Check sheet for the drawn part. Datum: minimum x, y, z corner. Units: mm. Round coordinates to 2 decimals unless told otherwise and drop trailing zeros. Write each loop counter-clockwise with the first axis right and the second up, starting at its lowest first coordinate (ties: lowest second). Pieces come first, ordered by that corner, then holes.
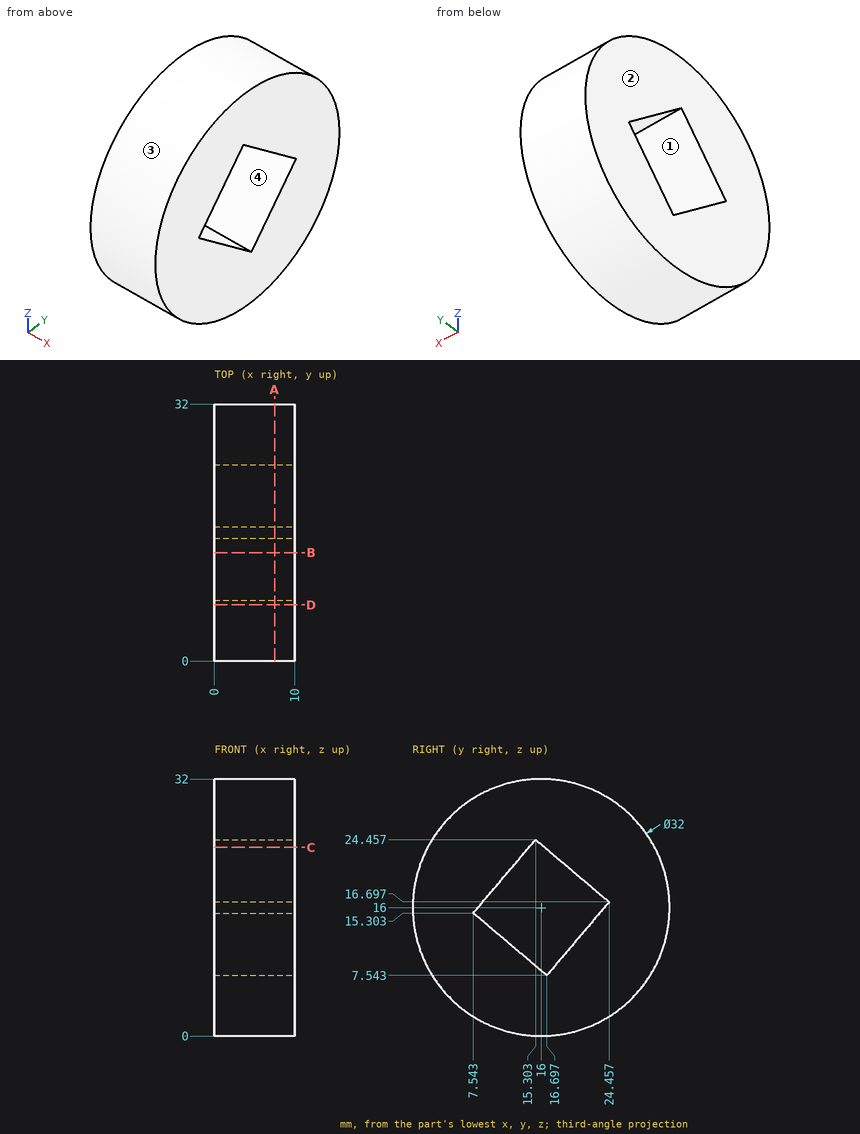
Q1. Sectioned sample at B-B (y = 13.5). Enter the section's corners in (x, z), plus the area to 3 significant figures.
Recorded:
outline: (0, 0.2) - (10, 0.2) - (10, 10.25) - (0, 10.25) - close; (0, 22.33) - (10, 22.33) - (10, 31.8) - (0, 31.8) - close
area: 195 mm2
Q2. Depth check by flat-ended pin: P1, Ø1.5, axis at x = 6.5, z = 10, coming from the +Y side; P2, Ø4, axis at x = 9, z = 12.5, coming from the -Y side; P3, Ø3, axis at x = 1.5, y = 23.5, coming from the +Z side; P4, Ø1, axis at y = 14.5, z = 11.5, coming from the +X side. Enter the tip coordinate at first touch or a pass-through.
Recorded:
P1: stops at y = 31.11
P2: stops at y = 0.07
P3: stops at z = 30.83
P4: passes through
Q3. Sectioned sample at A-A (x = 7.5). Enter the section's corners in (y, z).
Recorded:
outline: circle Ø32 at (16, 16); hole (7.54, 15.3) - (16.7, 7.54) - (24.46, 16.7) - (15.3, 24.46) - close
Q4. Release check for a two-part mould opening along Z. For the marked faces 1, 2, 3 and 4 record: released by +Z, released by -Z, zero draft, split by the parting line, or undercut.
Recorded:
face 1: undercut
face 2: zero draft
face 3: split by the parting line
face 4: undercut
Q5. Material ranges on line 1 along Y through (x, z) = (5.5, 13.5) (1 decimal); line 2 along Y through (x, z) = (4.75, 16.5); line 3 along Z through (x, y) = (8, 23) (1 decimal), recorded low to high.
Recorded:
line 1: y = 0.2 to 9.7, 21.7 to 31.8
line 2: y = 0.01 to 8.56, 24.29 to 31.99
line 3: z = 1.6 to 15, 17.9 to 30.4
Q6. Sectioned sample at C-C (z = 23.5). Enter the section's corners in (x, y), plus the area to 3 significant figures.
Recorded:
outline: (0, 1.87) - (10, 1.87) - (10, 14.49) - (0, 14.49) - close; (0, 16.43) - (10, 16.43) - (10, 30.13) - (0, 30.13) - close
area: 263 mm2
Q7. Sectioned sample at D-D (y = 7). Enter the section's corners in (x, z).
Recorded:
outline: (0, 2.77) - (10, 2.77) - (10, 29.23) - (0, 29.23) - close
